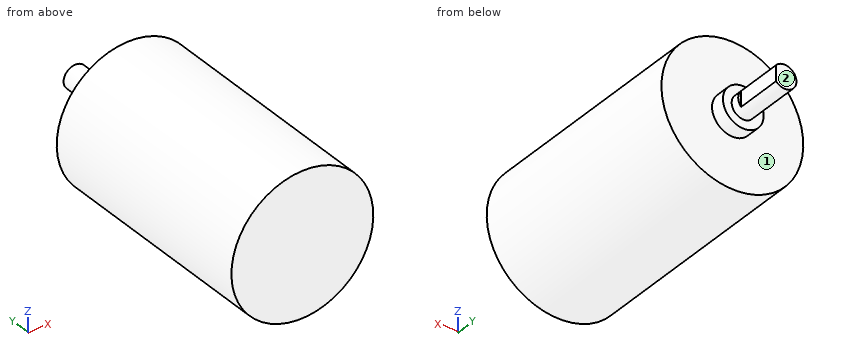
```python
from build123d import *

# Parameters (mm, degrees)
SKETCH1_R           = 12.2
BOSS_EXTRUDE1_DEPTH = 40
SKETCH2_R           = 3.5
BOSS_EXTRUDE2_DEPTH = 2.5
SKETCH3_R           = 2
BOSS_EXTRUDE3_DEPTH = 9.5
SKETCH4_W           = 1
SKETCH4_H           = 4
CUT_EXTRUDE1_DEPTH  = 8


with BuildPart() as part:
    # Sketch1 → Boss-Extrude1 (new body)
    with BuildSketch(Plane(origin=(0, 0, 0), x_dir=(1, 0, 0), z_dir=(0, 1, 0))):
        with Locations(Location((0, 0, 0), (0, 0, 270))):
            Circle(SKETCH1_R)
    extrude(amount=BOSS_EXTRUDE1_DEPTH)

    # Sketch2 → Boss-Extrude2 (add)
    with BuildSketch(Plane(origin=(0, 40, 0), x_dir=(1, 0, 0), z_dir=(0, 1, 0))):
        with Locations(Location((0, 0, 0), (0, 0, 270))):
            Circle(SKETCH2_R)
    extrude(amount=BOSS_EXTRUDE2_DEPTH)

    # Sketch3 → Boss-Extrude3 (add)
    with BuildSketch(Plane(origin=(0, 42.5, 0), x_dir=(1, 0, 0), z_dir=(0, 1, 0))):
        with Locations(Location((0, 0, 0), (0, 0, 270))):
            Circle(SKETCH3_R)
    extrude(amount=BOSS_EXTRUDE3_DEPTH)

    # Sketch4 → Cut-Extrude1 (cut)
    with BuildSketch(Plane(origin=(0, 52, 0), x_dir=(1, 0, 0), z_dir=(0, 1, 0))):
        with Locations((2, 0)):
            Rectangle(SKETCH4_W, SKETCH4_H)
    extrude(amount=-CUT_EXTRUDE1_DEPTH, mode=Mode.SUBTRACT)


solid = part.part
```
Verification items for the finished model (mm, model axes). Face numbers are marked on the shaded views. A direction names the side the tool comes from. Give positions to 0.01 mm unless a question says otherwise; leave off trailing zeros. Order: outer loops, then holes, each group sorted by start corner. A loop starts at its lowest first (then second) coordinate and runs counter-clockwise, first axis right, second up. Notation, with made-up numbers: (42, -7) -> (91, -7) arc R10 cw to (91, 7) -> close; hole circle Ø4 at (43.5, 33.25). An arc over 180 degrees is marked (long way). Use a Markdown table: item, result.
1) Material ranges on probe 1 along Y at (x, z) = (8, -2.5); probe 2 along X at (y, z) = (9, 0.25); probe 3 along Z at (x, y) = (10.5, 23), recorded low to high.
Results:
| item | result |
|---|---|
| probe 1 | 0 to 40 |
| probe 2 | -12.2 to 12.2 |
| probe 3 | -6.21 to 6.21 |
2) Section check C-C, the plane y = 26.5. Record the boundary of the cut face in (x, z), then the cut area to 3 significant figures.
Results:
| item | result |
|---|---|
| outline | circle Ø24.4 at (0, 0) |
| area | 468 mm² |
3) Tool access check on the marked faces 1 and 2. Record the directions out of +Z, -Z, +X, -X, +Y, -Y that give a thin tool (end or side, any length) a straight path to the whole face; none if there is none.
Results:
| item | result |
|---|---|
| face 1 | +Y |
| face 2 | +Z, -Z, +X, -X, +Y |
4) Section check B-B, the plane z = 0. Record the boundary of the cut face in (x, y).
Results:
| item | result |
|---|---|
| outline | (-12.2, 0) -> (12.2, 0) -> (12.2, 40) -> (3.5, 40) -> (3.5, 42.5) -> (2, 42.5) -> (2, 44) -> (1.5, 44) -> (1.5, 52) -> (-2, 52) -> (-2, 42.5) -> (-3.5, 42.5) -> (-3.5, 40) -> (-12.2, 40) -> close |
5) Section check D-D, the plane x = -2.75. Record the boundary of the cut face in (y, z).
Results:
| item | result |
|---|---|
| outline | (0, -11.89) -> (40, -11.89) -> (40, -2.17) -> (42.5, -2.17) -> (42.5, 2.17) -> (40, 2.17) -> (40, 11.89) -> (0, 11.89) -> close |
6) Depth check by flat-ended pin: pin 1 Ø4 at (y, z) = (23.5, -6.5) entering from +X; pin 2 Ø4 at (x, y) = (2.5, 15) entering from -Z; pin 3 Ø4 at (x, y) = (-4.5, 28) entering from -Z. Enter the tip coordinate at first touch or a pass-through.
Results:
| item | result |
|---|---|
| pin 1 | x = 11.34 |
| pin 2 | z = -12.19 |
| pin 3 | z = -11.94 |
7) Section check A-A, the plane x = 0. Record the boundary of the cut face in (y, z).
Results:
| item | result |
|---|---|
| outline | (0, -12.2) -> (40, -12.2) -> (40, -3.5) -> (42.5, -3.5) -> (42.5, -2) -> (52, -2) -> (52, 2) -> (42.5, 2) -> (42.5, 3.5) -> (40, 3.5) -> (40, 12.2) -> (0, 12.2) -> close |
